The model under review builds one solid part; all positions refer to its coordinate system, in mm. A direction names the side the tool comes from. Give positions to 0.01 mm unless a question says otherwise; leave off trailing zeros. Order: outer loops, then holes, each group sorted by start corner. A loop starts at its lowest first (then second) coordinate and runs counter-clockwise, first axis right, second up.
```python
from build123d import *

# Parameters (mm, degrees)
BOSS_EXTRU_1_START      = -10
ESQUISSE1_R             = 1
BOSS_EXTRU_1_DEPTH      = 10
BOSS_EXTRU_4_DEPTH      = 4
ESQUISSE3_R             = 1
ENL_V_MAT_EXTRU_1_DEPTH = 109.372369122


with BuildPart() as part:
    # Esquisse1 → Boss.-Extru.1 (new body)
    with BuildSketch(Plane.XY.offset(BOSS_EXTRU_1_START)):
        with BuildLine():
            add(Edge.make_bspline(
                [(18.84048499, -50.262173902), (59.909901441, -86.844998182), (76.538457933, -68.177081613)],
                knots=[4.71238898, 4.71238898, 4.71238898, 6.283185307, 6.283185307, 6.283185307], degree=2, weights=[1, 0.707106781, 1]))
            add(Edge.make_bspline(
                [(76.538457933, -68.177081613), (93.167014424, -49.509165044), (52.097597972, -12.926340764)],
                knots=[0, 0, 0, 1.570796327, 1.570796327, 1.570796327], degree=2, weights=[1, 0.707106781, 1]))
            Line((52.097597972, -12.926340764), (16.628556491, 18.667916569))
            ThreePointArc((16.628556491, 18.667916569), (-18.667916569, 16.628556491), (-16.628556491, -18.667916569))
            Line((-16.628556491, -18.667916569), (18.84048499, -50.262173902))
        make_face()
        with Locations((72.804874619, -64.851370315)):
            Circle(ESQUISSE1_R, mode=Mode.SUBTRACT)
    extrude(amount=-BOSS_EXTRU_1_DEPTH)

    # Esquisse2 → Boss.-Extru.4 (add)
    with BuildSketch(Plane(origin=(0, 0, -20), x_dir=(-1, 0, 0), z_dir=(0, 0, -1))):
        with BuildLine():
            Line((-23.527848394, -14.931187158), (-30.51184212, -7.090662199))
            ThreePointArc((-30.51184212, -7.090662199), (-35.509733497, -17.426184936), (-31.735458167, -28.268546035))
            Line((-31.735458167, -28.268546035), (-23.894933208, -21.284552309))
            ThreePointArc((-23.894933208, -21.284552309), (-25.027215807, -18.031843979), (-23.527848394, -14.931187158))
        make_face()
        with BuildLine():
            ThreePointArc((-31.735458167, -28.268546035), (-21.39993543, -33.266437412), (-10.557574331, -29.492162082))
            Line((-10.557574331, -29.492162082), (-17.541568057, -21.651637123))
            ThreePointArc((-17.541568057, -21.651637123), (-20.794276387, -22.783919722), (-23.894933208, -21.284552309))
            Line((-23.894933208, -21.284552309), (-31.735458167, -28.268546035))
        make_face()
        with BuildLine():
            Line((-23.527848394, -14.931187158), (-30.51184212, -7.090662199))
            ThreePointArc((-30.51184212, -7.090662199), (-35.509733497, -17.426184936), (-31.735458167, -28.268546035))
            Line((-31.735458167, -28.268546035), (-23.894933208, -21.284552309))
            ThreePointArc((-23.894933208, -21.284552309), (-25.027215807, -18.031843979), (-23.527848394, -14.931187158))
        make_face()
        with BuildLine():
            ThreePointArc((-31.735458167, -28.268546035), (-21.39993543, -33.266437412), (-10.557574331, -29.492162082))
            Line((-10.557574331, -29.492162082), (-17.541568057, -21.651637123))
            ThreePointArc((-17.541568057, -21.651637123), (-20.794276387, -22.783919722), (-23.894933208, -21.284552309))
            Line((-23.894933208, -21.284552309), (-31.735458167, -28.268546035))
        make_face()
        with BuildLine():
            ThreePointArc((-14.254741883, -4.669296932), (-22.744462605, -3.455072107), (-30.51184212, -7.090662199))
            Line((-30.51184212, -7.090662199), (-23.527848394, -14.931187158))
            Line((-23.527848394, -14.931187158), (-14.166195215, -4.931421004))
            ThreePointArc((-14.166195215, -4.931421004), (-14.211072924, -4.800563129), (-14.254741883, -4.669296932))
        make_face()
        with BuildLine():
            Line((-17.541568057, -21.651637123), (-10.557574331, -29.492162082))
            ThreePointArc((-10.557574331, -29.492162082), (-6.847907862, -24.429123097), (-5.534708226, -18.29141214))
            ThreePointArc((-5.534708226, -18.29141214), (-5.722194458, -15.927213359), (-6.279966343, -13.622115208))
            ThreePointArc((-6.279966343, -13.622115208), (-6.405329622, -13.563618707), (-6.530148083, -13.503968528))
            Line((-6.530148083, -13.503968528), (-17.541568057, -21.651637123))
        make_face()
        with BuildLine():
            ThreePointArc((-5.522244788, 4.301722039), (-5.110106455, 4.784016306), (-4.655995817, 5.227016639))
            Line((-4.655995817, 5.227016639), (-9.977133895, 11.200749941))
            ThreePointArc((-9.977133895, 11.200749941), (-14.483112506, 3.903774088), (-14.254741883, -4.669296932))
            ThreePointArc((-14.254741883, -4.669296932), (-14.138662596, -4.723413014), (-14.023049593, -4.778518229))
            Line((-14.023049593, -4.778518229), (-5.522244788, 4.301722039))
        make_face()
        with BuildLine():
            Line((-9.977133895, 11.200749941), (-4.655995817, 5.227016639))
            ThreePointArc((-4.655995817, 5.227016639), (2.864265113, 6.387173503), (7, 0))
            ThreePointArc((7, 0), (6.387173503, -2.864265113), (4.655995817, -5.227016639))
            Line((4.655995817, -5.227016639), (9.977133895, -11.200749941))
            ThreePointArc((9.977133895, -11.200749941), (13.686800364, -6.137710957), (15, 0))
            ThreePointArc((15, 0), (6.137710957, 13.686800364), (-9.977133895, 11.200749941))
        make_face()
        with BuildLine():
            Line((9.977133895, -11.200749941), (4.655995817, -5.227016639))
            ThreePointArc((4.655995817, -5.227016639), (4.163642753, -5.627084416), (3.637091246, -5.980933645))
            Line((3.637091246, -5.980933645), (-6.361776479, -13.379385501))
            ThreePointArc((-6.361776479, -13.379385501), (-6.320353283, -13.500575724), (-6.279966343, -13.622115208))
            ThreePointArc((-6.279966343, -13.622115208), (2.209754379, -14.836340033), (9.977133895, -11.200749941))
        make_face()
        with BuildLine():
            Line((-10.557574331, -29.492162082), (9.977133895, -11.200749941))
            ThreePointArc((9.977133895, -11.200749941), (2.209754379, -14.836340033), (-6.279966343, -13.622115208))
            ThreePointArc((-6.279966343, -13.622115208), (-5.722194458, -15.927213359), (-5.534708226, -18.29141214))
            ThreePointArc((-5.534708226, -18.29141214), (-6.847907862, -24.429123097), (-10.557574331, -29.492162082))
        make_face()
        with BuildLine():
            ThreePointArc((-14.254741883, -4.669296932), (-14.483112506, 3.903774088), (-9.977133895, 11.200749941))
            Line((-9.977133895, 11.200749941), (-30.51184212, -7.090662199))
            ThreePointArc((-30.51184212, -7.090662199), (-22.744462605, -3.455072107), (-14.254741883, -4.669296932))
        make_face()
    extrude(amount=BOSS_EXTRU_4_DEPTH)

    # Esquisse3 → Enlèv. mat.-Extru.1 (cut, through all)
    with BuildSketch(Plane(origin=(0, 0, -20), x_dir=(-1, 0, 0), z_dir=(0, 0, -1))):
        with Locations((-20.036872227, -17.847961796)):
            Circle(ESQUISSE3_R)
        with Locations((-22.028141551, -19.621696659)):
            Circle(ESQUISSE3_R)
        with Locations((-18.045602902, -16.074226932)):
            Circle(ESQUISSE3_R)
        with Locations((-16.054333578, -14.300492068)):
            Circle(ESQUISSE3_R)
        with Locations((-14.063064253, -12.526757204)):
            Circle(ESQUISSE3_R)
        with Locations((-12.071794928, -10.753022341)):
            Circle(ESQUISSE3_R)
    extrude(amount=-ENL_V_MAT_EXTRU_1_DEPTH, mode=Mode.SUBTRACT)


solid = part.part
```
Item 1: Draft analysis for pull direction Y (two halves, no side actions). For faces 6 (the flat face through (11.96, -17.52, -21.97)), 7 (the flat face through (34.61, 2.65, -14.93)), 8 (the cylindrical face through (-18.298, 17.035, -14.93)), state which applies: released by +Y, released by -Y, zero draft, split by the parting line, or undercut.
Values found:
face 6: undercut
face 7: released by +Y
face 8: split by the parting line
Item 2: For faces 1 (the flat face through (1.292, -9.628, -21.972)), 2 (the flat face through (20.101, 2.183, -21.972)), 3 (the flat face through (0.43, -20.47, -21.97)), 4 (the flat face through (33, -30, -10)), 5 (the flat face through (5, -14, -24)), list the 3-axis set-ups (+Z, -Z, +X, -X, +Y, -Y) from which the entire face can be reached by the end or side of a thin tool; tool diameter is ignored.
Values found:
face 1: -Z
face 2: -Z, +X, +Y
face 3: -Z, -X, -Y
face 4: +Z, +X, -X, +Y, -Y
face 5: -Z, +X, -X, +Y, -Y
Item 3: Take a section at C-C (z = -14). Give the number of separate pieces and of enclosed holes in the cut face, and give its area (3 significant figures).
Values found:
separate pieces: 1
enclosed holes: 7
area: 5,490 mm2
Item 4: Clearance check with flat-ended pins moving along their axes: pin 1 Ø4 at (x, z) = (59, -14) entering from +Y (3 decimals); pin 2 Ø6 at (x, z) = (59.5, -21) entering from -Y; pin 3 Ø8 at (x, y) = (55, -57.5) entering from -Z; pin 4 Ø1.6 at (x, y) = (16.05, -14.3) entering from +Z. State where each tip first meets the part, or that it passes through.
Values found:
pin 1: stops at y = -17.545
pin 2: stops at y = -72.58
pin 3: stops at z = -20
pin 4: passes through
Item 5: Take a section at B-B (x = 0). Give the boundary of the cut face in (y, z), and give its area (3 significant figures).
Values found:
outline: (-33.48, -20) - (-20.09, -20) - (-20.09, -24) - (-8.67, -24) - (-8.67, -20) - (7, -20) - (7, -24) - (15, -24) - (15, -20) - (25, -20) - (25, -10) - (-33.48, -10) - close
area: 662 mm2
Item 6: For line 1 (Z direction, x = 42, y = -42); line 2 (Y direction, x = -10, z = -22.75); line 3 (Y direction, x = 14.5, z = -14.5), list the stretches that pass through material, from the lowest coordinate up.
Values found:
line 1: z = -20 to -10
line 2: y = -11.18 to 11.18
line 3: y = -46.4 to -13.43, -11.63 to 20.37
